```python
from build123d import *

# Parameters (mm, degrees)
SKETCH1_R           = 1.1
SKETCH1_R_2         = 1.2
BOSS_EXTRUDE1_DEPTH = 2
SKETCH2_4_R         = 1.2
SKETCH2_4_R_2       = 2.083333333
SKETCH2_4_R_3       = 2.1
SKETCH2_4_R_4       = 1.1
BOSS_EXTRUDE2_DEPTH = 0.6


with BuildPart() as part:
    # Sketch1 → Boss-Extrude1 (new body)
    with BuildSketch(Plane(origin=(0, 0, 0), x_dir=(1, 0, 0), z_dir=(0, 1, 0))):
        with BuildLine():
            Line((-11.916666667, 1.054220702), (-11.916666667, -8.554220702))
            ThreePointArc((-11.916666667, -8.554220702), (-12.419965446, -10.571901894), (-10.927318432, -12.019780323))
            Line((-10.927318432, -12.019780323), (-8.048319684, -16.65121309))
            Line((-8.048319684, -16.65121309), (-1.895755615, -18.903388425))
            ThreePointArc((-1.895755615, -18.903388425), (0, -20.1), (1.895755615, -18.903388425))
            Line((1.895755615, -18.903388425), (8.048319684, -16.65121309))
            Line((8.048319684, -16.65121309), (10.927318432, -12.019780323))
            ThreePointArc((10.927318432, -12.019780323), (12.419965446, -10.571901894), (11.916666667, -8.554220702))
            Line((11.916666667, -8.554220702), (11.916666667, 1.054220702))
            ThreePointArc((11.916666667, 1.054220702), (12.416732246, 3.083108444), (10.904671205, 4.52537141))
            Line((10.904671205, 4.52537141), (5.822800045, 12.5))
            Line((5.822800045, 12.5), (-5.822800045, 12.5))
            Line((-5.822800045, 12.5), (-10.904671205, 4.52537141))
            ThreePointArc((-10.904671205, 4.52537141), (-12.416732246, 3.083108444), (-11.916666667, 1.054220702))
        make_face()
        with BuildLine():
            Line((8.333333333, 0.601446463), (8.333333333, 2.5))
            ThreePointArc((8.333333333, 2.5), (8.484662813, 1.720488044), (8.916666667, 1.054220702))
            Line((8.916666667, 1.054220702), (8.916666667, 0))
            Line((8.916666667, 0), (8.333333333, 0.601446463))
        make_face(mode=Mode.SUBTRACT)
        with Locations((0, -18)):
            Circle(SKETCH1_R, mode=Mode.SUBTRACT)
        with Locations((-10.416666667, -10)):
            Circle(SKETCH1_R_2, mode=Mode.SUBTRACT)
        with BuildLine():
            Line((-0.864511388, -16.086202712), (-4.970097661, -14.583333333))
            Line((-4.970097661, -14.583333333), (4.970097661, -14.583333333))
            Line((4.970097661, -14.583333333), (0.864511388, -16.086202712))
            ThreePointArc((0.864511388, -16.086202712), (0, -15.9), (-0.864511388, -16.086202712))
        make_face(mode=Mode.SUBTRACT)
        with Locations((10.416666667, -10)):
            Circle(SKETCH1_R_2, mode=Mode.SUBTRACT)
        with BuildLine():
            Line((-8.333333333, 0.601446463), (-8.916666667, -0.009018653))
            Line((-8.916666667, -0.009018653), (-8.916666667, 1.054220702))
            ThreePointArc((-8.916666667, 1.054220702), (-8.484662813, 1.720488044), (-8.333333333, 2.5))
            Line((-8.333333333, 2.5), (-8.333333333, 0.601446463))
        make_face(mode=Mode.SUBTRACT)
        with BuildLine():
            ThreePointArc((8.916666667, -8.554220702), (8.413367887, -9.428098106), (8.379462456, -10.435977959))
            Line((8.379462456, -10.435977959), (7.666241548, -11.583333333))
            Line((7.666241548, -11.583333333), (-7.666241548, -11.583333333))
            Line((-7.666241548, -11.583333333), (-8.379462456, -10.435977959))
            ThreePointArc((-8.379462456, -10.435977959), (-8.413367887, -9.428098106), (-8.916666667, -8.554220702))
            Line((-8.916666667, -8.554220702), (-8.916666667, -4.351446463))
            Line((-8.916666667, -4.351446463), (-5.333333333, -0.601446463))
            Line((-5.333333333, -0.601446463), (-5.333333333, 7.685759929))
            Line((-5.333333333, 7.685759929), (-4.177199955, 9.5))
            Line((-4.177199955, 9.5), (4.177199955, 9.5))
            Line((4.177199955, 9.5), (5.333333333, 7.685759929))
            Line((5.333333333, 7.685759929), (5.333333333, -0.601446463))
            Line((5.333333333, -0.601446463), (8.916666667, -4.351446463))
            Line((8.916666667, -4.351446463), (8.916666667, -8.554220702))
        make_face(mode=Mode.SUBTRACT)
        with Locations((-10.416666667, 2.5)):
            Circle(SKETCH1_R_2, mode=Mode.SUBTRACT)
        with Locations((10.416666667, 2.5)):
            Circle(SKETCH1_R_2, mode=Mode.SUBTRACT)
    extrude(amount=BOSS_EXTRUDE1_DEPTH)

    # Sketch2_4 → Boss-Extrude2 (add)
    with BuildSketch(Plane(origin=(0, 0, 0), x_dir=(1, 0, 0), z_dir=(0, 1, 0))):
        with BuildLine():
            ThreePointArc((-10.927318432, -12.019780323), (-8.614659909, -11.04549004), (-8.916666667, -8.554220702))
            ThreePointArc((-8.916666667, -8.554220702), (-12.218673424, -8.95450996), (-10.927318432, -12.019780323))
        make_face()
        with Locations((-10.416666667, -10)):
            Circle(SKETCH2_4_R, mode=Mode.SUBTRACT)
        with Locations((-10.416666667, 2.5)):
            Circle(SKETCH2_4_R_2)
        with Locations((-10.416666667, 2.5)):
            Circle(SKETCH2_4_R, mode=Mode.SUBTRACT)
        with BuildLine():
            ThreePointArc((8.916666667, -8.554220702), (8.614659909, -11.04549004), (10.927318432, -12.019780323))
            ThreePointArc((10.927318432, -12.019780323), (12.218673424, -8.95450996), (8.916666667, -8.554220702))
        make_face()
        with Locations((10.416666667, -10)):
            Circle(SKETCH2_4_R, mode=Mode.SUBTRACT)
        with Locations((0, -18)):
            Circle(SKETCH2_4_R_3)
        with Locations((0, -18)):
            Circle(SKETCH2_4_R_4, mode=Mode.SUBTRACT)
        with Locations((10.416666667, 2.5)):
            Circle(SKETCH2_4_R_2)
        with Locations((10.416666667, 2.5)):
            Circle(SKETCH2_4_R, mode=Mode.SUBTRACT)
    extrude(amount=-BOSS_EXTRUDE2_DEPTH)


solid = part.part
```
Geometry: final body of the model. Coordinates: model frame, mm. A direction names the side the tool comes from. Round coordinates to 2 decimals unless told otherwise and drop trailing zeros. Write each loop counter-clockwise with the first axis right and the second up, starting at its lowest first coordinate (ties: lowest second). Pieces come first, ordered by that corner, then holes. Notation, with made-up numbers: (-31.75, 7.25) -> (22.25, 7.25) arc R18 ccw to (22.25, 38.25) -> close; hole circle Ø3 at (87, 21.25). An arc over 180 degrees is marked (long way). Return JSON: item names as keys, results as strings.
Q1. Section A-A on z = 7.5. Return the cut outline in (x, y), and give its area (3 significant figures).
From the geometry:
{"outline": "(-11.92, 0) -> (-8.92, 0) -> (-8.92, 2) -> (-11.92, 2) -> close; (8.92, 0) -> (11.92, 0) -> (11.92, 2) -> (8.92, 2) -> close", "area": "12.0 mm2"}
Q2. Mould query, pull axis Z, two halves, no side actions, for faces 3 (the flat face through (8.917, 1, -0.5)), 4 (the flat face through (12, -0.6, 10)), 5 (the flat face through (0, 1, -12.5)), 6 (the flat face through (4.929, 0.986, 17.793)). Classes: +Z half, -Z half, draft (parallel to the pull), parting line (faces both ways), or undercut.
From the geometry:
{"face 3": "undercut", "face 4": "draft", "face 5": "-Z half", "face 6": "+Z half"}
Q3. Ray query, line 1 (X direction, y = 1.5, z = 10); line 2 (Z direction, x = 2, y = 1.3); line 3 (X direction, y = 1, z = -1). Return the intervals inside material, ascending.
From the geometry:
{"line 1": "-12.5 to -11.62, -9.22 to -8.33, 8.33 to 9.22, 11.62 to 12.5", "line 2": "-12.5 to -9.5, 11.58 to 14.58, 15.67 to 18.87", "line 3": "-11.92 to -8.92, -8.33 to -5.33, 5.33 to 8.33, 8.92 to 11.92"}
Q4. Section B-B on x = 2.75. Return the cut outline in (y, z).
From the geometry:
{"outline": "(0, -12.5) -> (2, -12.5) -> (2, -9.5) -> (0, -9.5) -> close; (0, 11.58) -> (2, 11.58) -> (2, 14.58) -> (0, 14.58) -> close; (0, 15.4) -> (2, 15.4) -> (2, 18.59) -> (0, 18.59) -> close"}
Q5. Section C-C on x = 0. Return the cut outline in (y, z), and give its area (3 significant figures).
From the geometry:
{"outline": "(-0.6, 15.9) -> (2, 15.9) -> (2, 16.9) -> (-0.6, 16.9) -> close; (-0.6, 19.1) -> (2, 19.1) -> (2, 20.1) -> (-0.6, 20.1) -> close; (0, -12.5) -> (2, -12.5) -> (2, -9.5) -> (0, -9.5) -> close; (0, 11.58) -> (2, 11.58) -> (2, 14.58) -> (0, 14.58) -> close", "area": "17.2 mm2"}
Q6. First-contact query: pin 1 Ø3 at (x, z) = (4, 14.5) entering from -Y; pin 2 Ø1 at (y, z) = (0.5, -9) entering from +X; pin 3 Ø1 at (y, z) = (1.5, -5.5) entering from -X. Flat tips, straight axial feed; report the tip coordinate or a pass-through.
From the geometry:
{"pin 1": "y = 0", "pin 2": "x = 8.37", "pin 3": "x = -10.6"}
Q7. Set-up query: faces 1 (the flat face through (7.1, 0.99, 2.45)), 2 (the flat face through (9.468, 0.986, 14.368)). Return all of +Z, -Z, +X, -X, +Y, -Y with unobstructed straight access to the full face (end or side cutting, diameter ignored); none if empty.
From the geometry:
{"face 1": "+Y, -Y", "face 2": "+Z, +X, +Y, -Y"}
Q8. Section D-D on z = 2. Return the cut outline in (x, y).
From the geometry:
{"outline": "(-11.92, 0) -> (-6.67, 0) -> (-6.67, 2) -> (-11.92, 2) -> close; (6.67, 0) -> (11.92, 0) -> (11.92, 2) -> (6.67, 2) -> close"}
